from build123d import *

# Parameters (mm, degrees)
SKETCH1_W               = 25.4
SKETCH1_H               = 38.1
BOSS_EXTRUDE1_DEPTH     = 1.5875
CUT_EXTRUDE1_DEPTH      = 41.192289761
CUT_EXTRUDE1_DEPTH_BACK = 41.192289761
SKETCH2_R               = 3.302
FILLET1_R               = 6.35


with BuildPart() as part:
    # Sketch1 → Boss-Extrude1 (new body)
    with BuildSketch(Plane.XY):
        with Locations((0, 19.05)):
            Rectangle(SKETCH1_W, SKETCH1_H)
    extrude(amount=BOSS_EXTRUDE1_DEPTH)

    # Sketch2 → Cut-Extrude1 (cut, two sides: drawn at the far end of the back side and taken through both)
    with BuildSketch(Plane.XY.offset(1.5875).offset(-CUT_EXTRUDE1_DEPTH_BACK)):
        with Locations((0, 25.4)):
            Circle(SKETCH2_R)
    extrude(amount=CUT_EXTRUDE1_DEPTH + CUT_EXTRUDE1_DEPTH_BACK, mode=Mode.SUBTRACT)

    # Fillet1
    fillet1_edges = [part.edges().sort_by_distance(p)[0] for p in [
        (-12.7, 38.1, 0.79375),
        (12.7, 38.1, 0.79375),
    ]]
    fillet(fillet1_edges, radius=FILLET1_R)


solid = part.part
Part model, mm, in its own coordinate system. Give positions to 0.01 mm unless a question says otherwise; leave off trailing zeros. Loops run counter-clockwise (first coordinate to the right, second up) from the corner with the lowest first, then second, coordinate; pieces in that order, holes last. Notation, with made-up numbers: (-16.75, 54.25) -> (10.25, 54.25) arc R20 cw to (10.25, 65.25) -> close; hole circle Ø9 at (83, 50). An arc over 180 degrees is marked (long way). Write each question's results on one line, items separated by ' | '. Start each with the question number.
Q1. Wall check: L1, parallel to X at y = 25.4, z = 1.1; L2, parallel to Y at x = 0, z = 1.1; L3, parallel to Y at x = -3, z = 1.45. Give the ranges that are in metal, low to high.
Q2. Pull direction Y, two halves, no side cores. Call faces 1 (the face through (-0.43, 28.674, 0.783)), 2 (the face through (0, 0, 1)), 3 (the face through (0, 19, 0)), 4 (the face through (0, 38.1, 1)): +Y half, -Y half, draft (parallel to the pull), parting line (faces both ways), or undercut.
Q3. Band-saw the part on A-A on y = 25.4. List the corners of the cut face in (x, z).
Q4. Band-saw the part on C-C on x = 0. List the corners of the cut face in (y, z).
Q5. Band-saw the part on B-B on z = 1.3. List the corners of the cut face in (x, y).
Results are:
1) L1: x = -12.7 to -3.3, 3.3 to 12.7 | L2: y = 0 to 22.1, 28.7 to 38.1 | L3: y = 0 to 24.02, 26.78 to 38.1
2) face 1: undercut | face 2: -Y half | face 3: draft | face 4: +Y half
3) outline: (-12.7, 0) -> (-3.3, 0) -> (-3.3, 1.59) -> (-12.7, 1.59) -> close; (3.3, 0) -> (12.7, 0) -> (12.7, 1.59) -> (3.3, 1.59) -> close
4) outline: (0, 0) -> (22.1, 0) -> (22.1, 1.59) -> (0, 1.59) -> close; (28.7, 0) -> (38.1, 0) -> (38.1, 1.59) -> (28.7, 1.59) -> close
5) outline: (-12.7, 0) -> (12.7, 0) -> (12.7, 31.75) arc R6.35 ccw to (6.35, 38.1) -> (-6.35, 38.1) arc R6.35 ccw to (-12.7, 31.75) -> close; hole circle Ø6.6 at (0, 25.4)
